Can you work these out from the drawing? Everything is in mm from the part's minimum corner. A direction names the side the tool comes from. Give positions to 0.01 mm unless a question says otherwise; leave off trailing zeros. Order: outer loops, then holes, each group sorted by start corner. A loop starts at its lowest first (then second) coordinate and runs counter-clockwise, first axis right, second up. Notation, with made-up numbers: (-10, -2) - (47, -2) arc R26 ccw to (47, 15) - close; hole circle Ø7 at (-5.75, 83). An arc over 180 degrees is marked (long way). One line per question, with ' | ' between items.
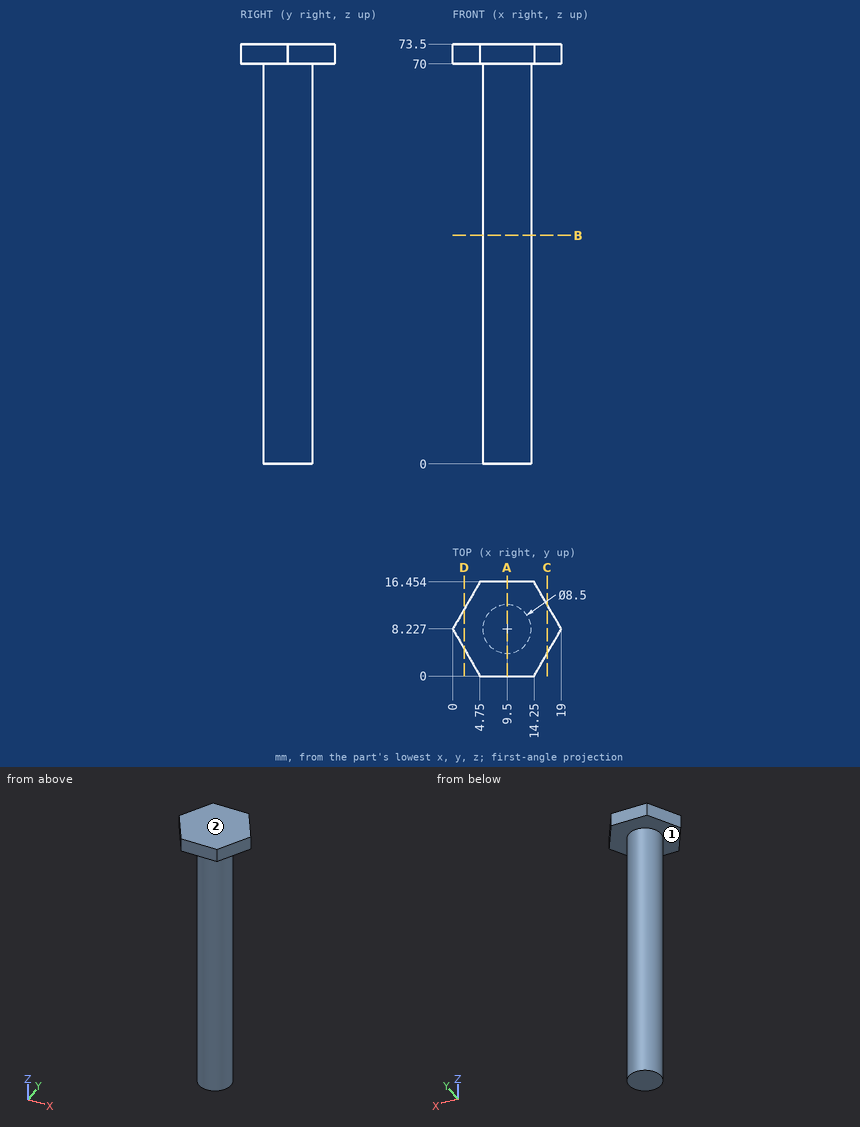
(1) Imagine slicing it at C-C (x = 16.5). List the corners of the cut face in (y, z) for me, and give its area (3 significant figures).
Answer below:
outline: (3.9, 70) - (12.56, 70) - (12.56, 73.5) - (3.9, 73.5) - close | area: 30.3 mm^2
(2) Imagine slicing it at A-A (x = 9.5). List the corners of the cut face in (y, z) for me (1 decimal).
Answer below:
outline: (0, 70) - (4, 70) - (4, 0) - (12.5, 0) - (12.5, 70) - (16.5, 70) - (16.5, 73.5) - (0, 73.5) - close
(3) If I drill on line 1 (Z direction, x = 14, y = 10.5); line 2 (Y direction, x = 6.25, z = 31) (1 decimal); line 3 (Y direction, x = 9.5, z = 24.5), over which ranges is the centre line in solid material (lowest first)?
Answer below:
line 1: 70 to 73.5 | line 2: 5.5 to 11 | line 3: 3.98 to 12.48
(4) Imagine slicing it at B-B (z = 40). List the corners of the cut face in (x, y) for me.
Answer below:
outline: circle Ø8.5 at (9.5, 8.23)
(5) Will these pins go through, and if not, where does the flat tip stop? pin 1 (1.5 mm diameter, centred on x = 13.5, z = 34.5, fed in from -Y); pin 2 (8 mm diameter, centred on x = 15.5, z = 52, fed in from -Y); pin 3 (4 mm diameter, centred on x = 13, z = 52, fed in from -Y).
Answer below:
pin 1: y = 5.49 | pin 2: y = 4.48 | pin 3: y = 4.25
(6) Imagine slicing it at D-D (x = 2). List the corners of the cut face in (y, z) for me.
Answer below:
outline: (4.76, 70) - (11.69, 70) - (11.69, 73.5) - (4.76, 73.5) - close
(7) On a 3-axis mill with a long thin cutter (end or side, diameter ignored), from which of +Z, -Z, +X, -X, +Y, -Y can I reach the whole of each face in a straight line? I mean the marked faces 1 and 2. Say none if no direction works.
Answer below:
face 1: -Z | face 2: +Z, +X, -X, +Y, -Y
